Autodesk Inventor part; units mm, degrees
ref_plane "YZ Plane" through (0, 0, 0) normal (1, 0, 0) x (0, 1, 0)
ref_plane "XZ Plane" through (0, 0, 0) normal (0, 1, 0) x (-1, 0, 0)
ref_plane "XY Plane" through (0, 0, 0) normal (0, 0, 1) x (1, 0, 0)
sketch "Sketch1" plane through (0, 0, 0) normal (0, 0, 1) x (1, 0, 0)
  line L0 (0, 0) -> (45, 0)
  line L1 (45, 0) -> (45, 20)
  line L2 (45, 20) -> (0, 20)
  line L3 (0, 20) -> (0, 0)
  circle A0 centre (6.5, 7) radius 2.75
  circle A1 centre (38.5, 7) radius 2.75
  dimension "d0" = 45
  dimension "d1" = 20
  dimension "d5" = 5.5
  dimension "d6" = 5.5
extrude "Extrusion1" add sketch "Sketch1" along normal blind 6
sketch "Sketch2" plane through (0, 0, 6) normal (0, 0, 1) x (1, 0, 0)
  line L0 (45, 20) -> (0, 20)
  line L1 (0, 20) -> (5, 20)
  line L2 (5, 20) -> (10, 20)
  line L3 (10, 20) -> (10, 14)
  line L4 (10, 14) -> (5, 14)
  line L5 (5, 14) -> (5, 20)
  point P0 (0, 0)
  dimension "d9" = 5
  dimension "d10" = 5
  dimension "d11" = 6
extrude "Extrusion2" cut sketch "Sketch2" against normal blind 6
pattern_linear "Rectangular Pattern1" count 4 spacing 10 along (1, 0, 0) of "Extrusion2"
properties part number "e_rail support"
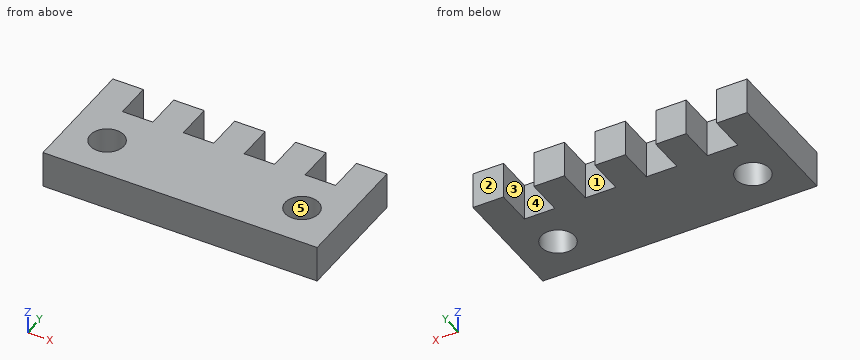
Geometry check sheet. Reference: the model listing, model coordinates, mm. Face numbers are marked on the shaded views. A direction names the side the tool comes from. Coordinates: 2 decimals unless noted, no trailing zeros. Loops run counter-clockwise (first coordinate to the right, second up) from the corner with the lowest first, then second, coordinate; pieces in that order, holes last. Notation, with made-up numbers: (17.5, 31) - (55.5, 31) arc R21 ccw to (55.5, 63) - close; hole circle Ø11 at (-19, 3). An arc over 180 degrees is marked (long way). One line per item, written item: value. Start each with the question number.
(1) Depth check by flat-ended pin: P1, Ø1.5, axis at x = 8, z = 4, coming from the +Y side. Enter the tip coordinate at first touch or a pass-through.
(2) Cross-section at C-C on z = 3.7. Enter the section's corners in (x, y).
(3) Cross-section at D-D on y = 17.75. Enter the section's corners in (x, z).
(4) Cross-section at A-A on x = 6.5. Enter the section's corners in (y, z), plus the area to 3 significant figures.
(5) Cross-section at B-B on y = 7. Enter the section's corners in (x, z).
(6) Material ranges on line 1 (Y direction, x = 38.5, z = 1.45); line 2 (X direction, y = 9.5, z = 2.05); line 3 (X direction, y = 15.25, z = 1.15), recorded low to high. Write a range as [from, to].
(7) Mould release check, pull along Y, two halves, no side actions. Record for the marked faces 3, 4 and 5: released by +Y, released by -Y, zero draft, split by the parting line, or undercut.
(8) Tool access check on the marked faces 1 and 2. Record the directions out of +Z, -Z, +X, -X, +Y, -Y that give a thin tool (end or side, any length) a straight path to the whole face; none if there is none.
Results below:
1. P1: stops at y = 14
2. outline: (0, 0) - (45, 0) - (45, 20) - (40, 20) - (40, 14) - (35, 14) - (35, 20) - (30, 20) - (30, 14) - (25, 14) - (25, 20) - (20, 20) - (20, 14) - (15, 14) - (15, 20) - (10, 20) - (10, 14) - (5, 14) - (5, 20) - (0, 20) - close; hole circle Ø5.5 at (6.5, 7); hole circle Ø5.5 at (38.5, 7)
3. outline: (0, 0) - (5, 0) - (5, 6) - (0, 6) - close; (10, 0) - (15, 0) - (15, 6) - (10, 6) - close; (20, 0) - (25, 0) - (25, 6) - (20, 6) - close; (30, 0) - (35, 0) - (35, 6) - (30, 6) - close; (40, 0) - (45, 0) - (45, 6) - (40, 6) - close
4. outline: (0, 0) - (4.25, 0) - (4.25, 6) - (0, 6) - close; (9.75, 0) - (14, 0) - (14, 6) - (9.75, 6) - close
4. area: 51.0 mm2
5. outline: (0, 0) - (3.75, 0) - (3.75, 6) - (0, 6) - close; (9.25, 0) - (35.75, 0) - (35.75, 6) - (9.25, 6) - close; (41.25, 0) - (45, 0) - (45, 6) - (41.25, 6) - close
6. line 1: y = [0, 4.25], [9.75, 14]
6. line 2: x = [0, 5.35], [7.65, 37.35], [39.65, 45]
6. line 3: x = [0, 5], [10, 15], [20, 25], [30, 35], [40, 45]
7. face 3: zero draft
7. face 4: released by +Y
7. face 5: undercut
8. face 1: +Z, -Z, +Y
8. face 2: +Z, -Z, +X, -X, +Y
